Verification items for this drawing (mm, ordinates from the low corner). A direction names the side the tool comes from. Coordinates: 2 decimals unless noted, no trailing zeros. Write each loop counter-clockwise with the first axis right and the second up, starting at its lowest first coordinate (ties: lowest second). Pieces come first, ordered by that corner, then holes.
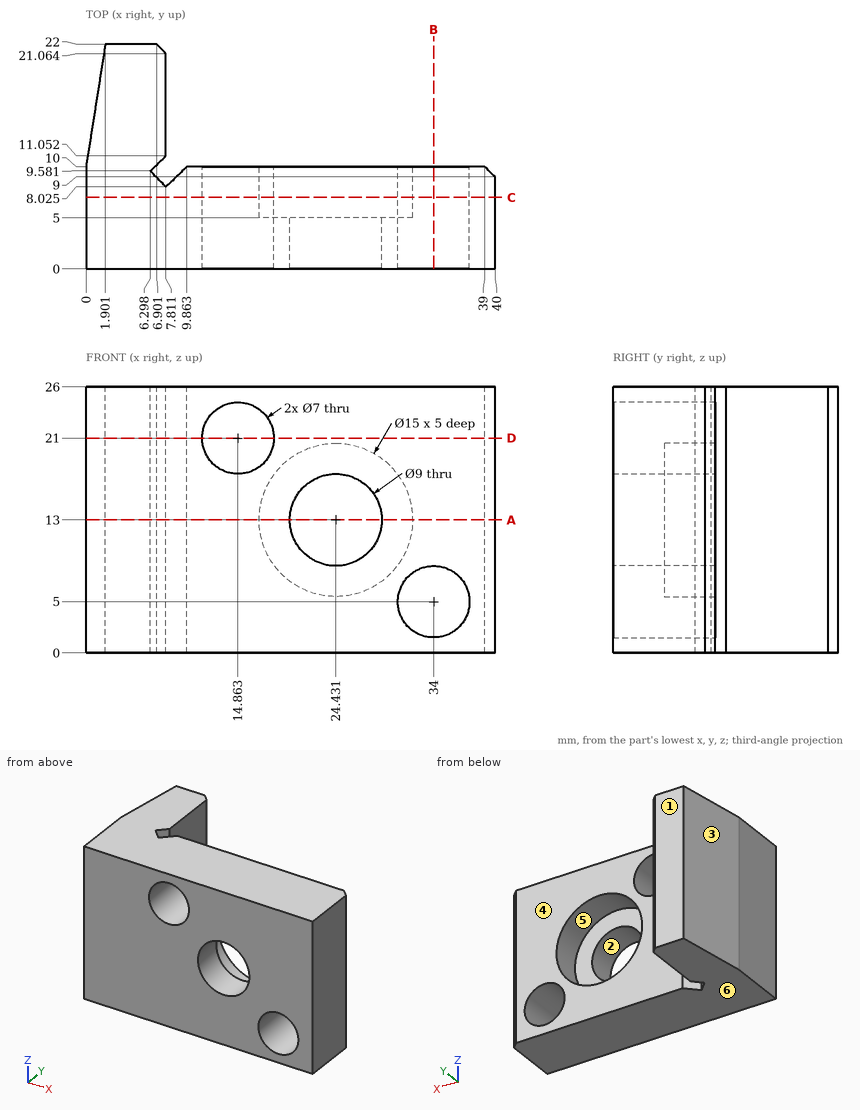
1. Sectioned sample at D-D, the plane z = 21. Record the boundary of the cut face in (x, y) (1 decimal).
Computed values:
outline: (0, 0) - (11.4, 0) - (11.4, 10) - (9.9, 10) - (7.8, 8) - (6.3, 9.6) - (7.8, 11.1) - (7.8, 21.1) - (6.9, 22) - (1.9, 22) - (0, 10) - close; (18.4, 0) - (40, 0) - (40, 9) - (39, 10) - (18.4, 10) - close
2. Gauge pin test, flat ends, axial feed: pin 1 Ø12 at (y, z) = (17.5, 23) entering from +X; pin 2 Ø5.5 at (x, z) = (34, 5) entering from -Y; pin 3 Ø14.5 at (x, z) = (24.43, 13) entering from +Y; pin 4 Ø2 at (y, z) = (19.5, 21.5) entering from -X. Record the tip position at first contact, or that the pin passes through.
Computed values:
pin 1: stops at x = 7.81
pin 2: passes through
pin 3: stops at y = 5
pin 4: stops at x = 1.35
3. Access from +Z, -Z, +X, -X, +Y, -Y to the whole of each face (thin tool, end or side, straight path). Record for the marked faces 4, 5 and 6.
Computed values:
face 4: +Z, -Z, +X, +Y
face 5: +Y
face 6: -Z, +X, -X, +Y, -Y
4. Thickness scan on line 1 along X through (y, z) = (2.25, 5); line 2 along X through (y, z) = (2.25, 13); line 3 along Y through (x, z) = (15.5, 1.25). Record the ranges inside material, lowest first.
Computed values:
line 1: x = 0 to 30.5, 37.5 to 40
line 2: x = 0 to 19.93, 28.93 to 40
line 3: y = 0 to 10
5. Sectioned sample at C-C, the plane y = 7. Record the boundary of the cut face in (x, z).
Computed values:
outline: (0, 0) - (40, 0) - (40, 26) - (0, 26) - close; hole circle Ø7 at (14.86, 21); hole circle Ø15 at (24.43, 13); hole circle Ø7 at (34, 5)
6. Sectioned sample at A-A, the plane z = 13. Record the boundary of the cut face in (x, y) (1 decimal), and give its area (3 significant figures).
Computed values:
outline: (0, 0) - (19.9, 0) - (19.9, 5) - (16.9, 5) - (16.9, 10) - (9.9, 10) - (7.8, 8) - (6.3, 9.6) - (7.8, 11.1) - (7.8, 21.1) - (6.9, 22) - (1.9, 22) - (0, 10) - close; (28.9, 0) - (40, 0) - (40, 9) - (39, 10) - (31.9, 10) - (31.9, 5) - (28.9, 5) - close
area: 357 mm2
7. Draft check along X on the marked faces 1, 2 and 3. Enter one of: released by +X, released by -X, zero draft, split by the parting line, or undercut.
Computed values:
face 1: zero draft
face 2: undercut
face 3: released by -X
8. Sectioned sample at B-B, the plane x = 34. Record the boundary of the cut face in (y, z).
Computed values:
outline: (0, 0) - (10, 0) - (10, 1.5) - (0, 1.5) - close; (0, 8.5) - (10, 8.5) - (10, 26) - (0, 26) - close
